The model under review builds one solid part; all positions refer to its coordinate system, in mm. A direction names the side the tool comes from. Coordinates: 2 decimals unless noted, no trailing zeros. Order: outer loops, then holes, each group sorted by start corner. A loop starts at its lowest first (then second) coordinate and runs counter-clockwise, first axis right, second up. Notation, with made-up numbers: (-3, 1) -> (45, 1) arc R27 ccw to (45, 35) -> close; hole circle Ø8 at (-12.75, 45). An arc over 180 degrees is marked (long way). Use one line per item in the form item = value. Start each with the question number.
(1) Wall thickness on line 1 along X through (y, z) = (-35, 11); line 2 along Y through (x, z) = (126.1, 20); line 3 along X through (y, z) = (-34.5, 13): over which ranges is each line inside the solid? List them lowest first.
(2) Mouldability with a two-part tool opening along Y and no side actions: class faces 1 (the flat face through (89, -40, 20)), 2 (the flat face through (50, -37, 20)), 3 (the cylindrical face through (89.51, -33.81, 20.16)) as +Y half, -Y half, draft (parallel to the pull), parting line (faces both ways), or undercut.
(3) For faces 4 (the cylindrical face through (128.02, -33.99, 19.35)), 5 (the cylindrical face through (125.65, -33.99, 34.3)), list the 3-axis set-ups (+Z, -Z, +X, -X, +Y, -Y) from which the entire face can be reached by the end or side of a thin tool; tool diameter is ignored.
(4) Insertion check: pin 1 Ø2 at (x, y) = (125, -35) entering from -Z. The pin has a flat end and moves straight along its axis. Give the tip position at first contact, or say it passes through.
(5) Take a section at A-A (z = 33). State the section outline as (x, y) points.
(6) Take a section at B-B (y = -35). State the section outline as (x, z) points.
```python
from build123d import *

# Parameters (mm, degrees)
CYLINDER107_R     = 1.2
CYLINDER107_DEPTH = 100
CYLINDER110_R     = 1.2
CYLINDER110_DEPTH = 100
CYLINDER108_R     = 1.2
CYLINDER108_DEPTH = 100
BOX038_W          = 80
BOX038_H          = 10
BOX038_DEPTH      = 57
FILLET015_R       = 4


with BuildPart() as screwhole055:
    # Cylinder107 → Cylinder107 (new body)
    with BuildSketch(Plane(origin=(125, -35, -20), x_dir=(1, 0, 0), z_dir=(0, 0, 1))):
        Circle(CYLINDER107_R)
    extrude(amount=CYLINDER107_DEPTH)


with BuildPart() as screwhole058:
    # Cylinder110 → Cylinder110 (new body)
    with BuildSketch(Plane(origin=(55, -35, 20), x_dir=(0, 0, -1), z_dir=(1, 0, 0))):
        Circle(CYLINDER110_R)
    extrude(amount=CYLINDER110_DEPTH)


with BuildPart() as fusion001002012030037:
    # Cylinder108 → Cylinder108 (new body)
    with BuildSketch(Plane(origin=(55, -35, -20), x_dir=(1, 0, 0), z_dir=(0, 0, 1))):
        Circle(CYLINDER108_R)
    extrude(amount=CYLINDER108_DEPTH)

    # Fusion001002012030037: union ScrewHole055, ScrewHole058
    add(screwhole055.part)
    add(screwhole058.part)


with BuildPart() as side001:
    # Box038 → Box038 (new body)
    with BuildSketch(Plane(origin=(50, -40, -8), x_dir=(1, 0, 0), z_dir=(0, 0, 1))):
        with Locations((40, 5)):
            Rectangle(BOX038_W, BOX038_H)
    extrude(amount=BOX038_DEPTH)

    # Fillet015
    fillet015_edges = [side001.edges().sort_by_distance(p)[0] for p in [
        (50, -30, 20.5),
    ]]
    fillet(fillet015_edges, radius=FILLET015_R)

    # Cut015017007031: cut Fusion001002012030037
    add(fusion001002012030037.part, mode=Mode.SUBTRACT)


solid = side001.part
```
Findings:
q1.line_1 = 50 to 53.8, 56.2 to 123.8, 126.2 to 130
q1.line_2 = -40 to -36.2, -33.8 to -30
q1.line_3 = 50 to 53.91, 56.09 to 123.91, 126.09 to 130
q2.face_1 = -Y half
q2.face_2 = draft
q2.face_3 = undercut
q3.face_4 = +X
q3.face_5 = +Z, -Z
q4.pin_1 = through
q5.outline = (50, -40) -> (130, -40) -> (130, -30) -> (54, -30) arc R4 ccw to (50, -34) -> close; hole circle Ø2.4 at (55, -35); hole circle Ø2.4 at (125, -35)
q6.outline = (50, -8) -> (53.8, -8) -> (53.8, 49) -> (50, 49) -> close; (56.2, -8) -> (123.8, -8) -> (123.8, 18.8) -> (56.2, 18.8) -> close; (56.2, 21.2) -> (123.8, 21.2) -> (123.8, 49) -> (56.2, 49) -> close; (126.2, -8) -> (130, -8) -> (130, 18.8) -> (126.2, 18.8) -> close; (126.2, 21.2) -> (130, 21.2) -> (130, 49) -> (126.2, 49) -> close
